Print and shaded views of the part. All mm, measured from the part's lowest x, y and z. A direction names the side the tool comes from. Coordinates: 2 decimals unless noted, no trailing zeros. Order: outer loops, then holes, each group sorted by start corner. A loop starts at its lowest first (then second) coordinate and runs counter-clockwise, first axis right, second up.
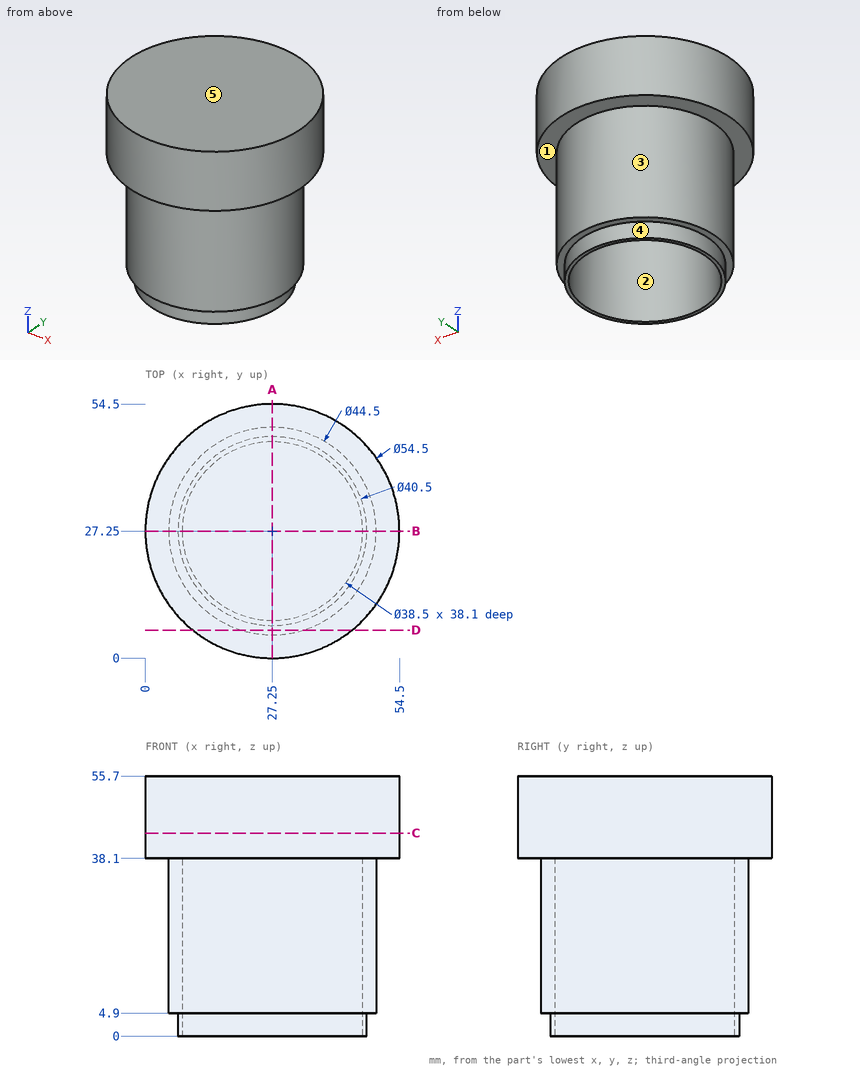
Q1. Cut at D-D, the plane y = 6. List the corners of the cut face in (x, z), plus the area to 3 significant figures.
Established:
outline: (10.19, 38.1) - (20.65, 38.1) - (20.65, 4.9) - (33.85, 4.9) - (33.85, 38.1) - (44.31, 38.1) - (44.31, 55.7) - (10.19, 55.7) - close
area: 1,040 mm2
Q2. Cut at A-A, the plane x = 27.25. List the corners of the cut face in (y, z).
Established:
outline: (0, 38.1) - (5, 38.1) - (5, 4.9) - (7, 4.9) - (7, 0) - (8, 0) - (8, 38.1) - (46.5, 38.1) - (46.5, 0) - (47.5, 0) - (47.5, 4.9) - (49.5, 4.9) - (49.5, 38.1) - (54.5, 38.1) - (54.5, 55.7) - (0, 55.7) - close
Q3. Drop flat-ended pins along their axis: P1, Ø13.5, axis at x = 32, y = 21, coming from the -Z side; P2, Ø1, axis at y = 30.5, z = 17, coming from the +X side; P3, Ø12, axis at y = 44.5, z = 34, coming from the -X side. Give the stop position or say it passes through.
Established:
P1: stops at z = 38.1
P2: stops at x = 49.33
P3: stops at x = 3.23
Q4. Which spindle directions (+Z, -Z, +X, -X, +Y, -Y) get a long thin tool onto all of the face, cutting with end or side? Do the marked faces 4 and 5. Say none if no direction does.
Established:
face 4: -Z
face 5: +Z, +X, -X, +Y, -Y
Q5. Mould opens along X. For the marked faces 1, 2 and 3 say: pulls with the +X half, pulls with the -X half, needs draft (parallel to the pull), parting line crosses it, or undercut.
Established:
face 1: needs draft
face 2: undercut
face 3: parting line crosses it
Q6. Probe line 1 (Y direction, x = 27, z = 20); line 2 (Z direction, x = 49, y = 33). List the from-to ranges inside material, lowest first.
Established:
line 1: y = 5 to 8, 46.5 to 49.5
line 2: z = 38.1 to 55.7
Q7. Cut at C-C, the plane z = 43.5. List the corners of the cut face in (x, y).
Established:
outline: circle Ø54.5 at (27.25, 27.25)
